from build123d import *

# Parameters (mm, degrees)
SKETCH1_W                    = 87
SKETCH1_H                    = 43
BASE_FLANGE1_DEPTH           = 2
EDGE_FLANGE1_STRIP_W         = 12
EDGE_FLANGE1_STRIP_H         = 2
EDGE_FLANGE1_STRIP_CUT_DEPTH = 87
EDGE_FLANGE1_DEPTH           = 87
CUT_EXTRUDE1_DEPTH           = 10


# Sheet-metal steps are written as plain solids
with BuildPart() as part:
    # Sketch1 → Base-Flange1 (new body)
    with BuildSketch(Plane(origin=(0, 0, 0), x_dir=(1, 0, 0), z_dir=(0, 1, 0))):
        Rectangle(SKETCH1_W, SKETCH1_H)
    extrude(amount=-BASE_FLANGE1_DEPTH)

    # Edge-Flange1 strip (across the edge) → Edge-Flange1 strip cut (cut)
    with BuildSketch(Plane(origin=(43.5, 0, -21.5), x_dir=(0, 0, 1), z_dir=(-1, 0, 0))):
        with Locations((-4, -1)):
            Rectangle(EDGE_FLANGE1_STRIP_W, EDGE_FLANGE1_STRIP_H)
    extrude(amount=EDGE_FLANGE1_STRIP_CUT_DEPTH, mode=Mode.SUBTRACT)

    # Edge-Flange1 section (across the edge) → Edge-Flange1 (add)
    with BuildSketch(Plane(origin=(43.5, 0, -21.5), x_dir=(0, 0, 1), z_dir=(-1, 0, 0))):
        with BuildLine():
            Line((-2, 2), (-2, 44))
            Line((-2, 44), (0, 44))
            Line((0, 44), (0, 2))
            ThreePointArc((0, 2), (0.585786438, 0.585786438), (2, 0))
            Line((2, 0), (2, -2))
            ThreePointArc((2, -2), (-0.828427125, -0.828427125), (-2, 2))
        make_face()
    extrude(amount=EDGE_FLANGE1_DEPTH)

    # Sketch9 → Cut-Extrude1 (cut)
    with BuildSketch(Plane(origin=(0, 0, -23.5), x_dir=(-1, 0, 0), z_dir=(0, 0, -1))):
        with BuildLine():
            Line((5.5, 28.548666546), (5.5, 15.848666546))
            ThreePointArc((5.5, 15.848666546), (0, 10.348666546), (-5.5, 15.848666546))
            Line((-5.5, 15.848666546), (-5.5, 28.548666546))
            ThreePointArc((-5.5, 28.548666546), (0, 34.048666546), (5.5, 28.548666546))
        make_face()
    extrude(amount=-CUT_EXTRUDE1_DEPTH, mode=Mode.SUBTRACT)


solid = part.part
Model file for the job. Use its own axes, mm. A direction names the side the tool comes from. Give positions to 0.01 mm unless a question says otherwise; leave off trailing zeros. Loops run counter-clockwise (first coordinate to the right, second up) from the corner with the lowest first, then second, coordinate; pieces in that order, holes last.
1) Flat gauge pins, fed straight in: pin 1 Ø12.5 at (x, y) = (-15, 26) entering from +Z; pin 2 Ø10 at (y, z) = (14.5, -19) entering from +X; pin 3 Ø12.5 at (x, z) = (-13.5, -2.5) entering from +Y; pin 4 Ø4 at (y, z) = (3.5, -11.5) entering from +X. Where does each tip first touch, or does it go through?
2) Saw through at B-B (x = 0). Write the cut outline in (y, z).
3) Wall check: line 1 (Z direction, x = -30.5, y = 20); line 2 (Y direction, x = 22.5, z = -17); line 3 (Z direction, x = 10.5, y = 1.5). Give the ranges that are in metal, low to high.
4) Saw through at C-C (x = -16). Write the cut outline in (y, z).
5) Tool access for faces 4 (the flat face through (-43.5, 11, -23)), 5 (the cylindrical face through (0.121, 34.047, -22.514)), 6 (the flat face through (10, 23, -21.5)): list every direction of +Z, -Z, +X, -X, +Y, -Y with a clear straight run to the whole face (end or side of a thin tool).
6) Pull direction X, two halves, no side cores. Call faces 1 (the flat face through (-1, -1, 21.5)), 2 (the flat face through (5.5, 22, -23)), 3 (the flat face through (43.5, 11, -23)): +X half, -X half, draft (parallel to the pull), parting line (faces both ways), or undercut.
7) Saw through at D-D (z = 5.5). Write the cut outline in (x, y), plus the area to 3 significant figures.
8) Saw through at A-A (y = 25.5). Write the cut outline in (x, z), plus the area to 3 significant figures.
Answer block:
1. pin 1: stops at z = -21.5
1. pin 2: stops at x = 43.5
1. pin 3: stops at y = 0
1. pin 4: passes through
2. outline: (-2, -19.5) arc R4 ccw to (2, -23.5) - (10.35, -23.5) - (10.35, -21.5) - (2, -21.5) arc R2 cw to (0, -19.5) - (0, 21.5) - (-2, 21.5) - close; (34.05, -23.5) - (44, -23.5) - (44, -21.5) - (34.05, -21.5) - close
3. line 1: z = -23.5 to -21.5
3. line 2: y = -2 to 0
3. line 3: z = -23.47 to -21.44
4. outline: (-2, -19.5) arc R4 ccw to (2, -23.5) - (44, -23.5) - (44, -21.5) - (2, -21.5) arc R2 cw to (0, -19.5) - (0, 21.5) - (-2, 21.5) - close
5. face 4: +Z, -Z, -X, +Y, -Y
5. face 5: +Z, -Z
5. face 6: +Z, +X, -X, +Y
6. face 1: draft
6. face 2: undercut
6. face 3: +X half
7. outline: (-43.5, -2) - (43.5, -2) - (43.5, 0) - (-43.5, 0) - close
7. area: 174 mm2
8. outline: (-43.5, -23.5) - (-5.5, -23.5) - (-5.5, -21.5) - (-43.5, -21.5) - close; (5.5, -23.5) - (43.5, -23.5) - (43.5, -21.5) - (5.5, -21.5) - close
8. area: 152 mm2
